from build123d import *

# Parameters (mm, degrees)
BOSS_EXTRUDE1_DEPTH = 97
FILLET1_R           = 3
SKETCH2_W           = 12.4
SKETCH2_H           = 5
CUT_EXTRUDE1_DEPTH  = 10


with BuildPart() as part:
    # Sketch1 → Boss-Extrude1 (new body)
    with BuildSketch(Plane(origin=(0, 0, 0), x_dir=(1, 0, 0), z_dir=(0, 1, 0))):
        with BuildLine():
            Line((-30, 11.1), (30, 11.1))
            ThreePointArc((30, 11.1), (37.071067812, 8.171067812), (40, 1.1))
            Line((40, 1.1), (40, -1.1))
            ThreePointArc((40, -1.1), (37.071067812, -8.171067812), (30, -11.1))
            Line((30, -11.1), (-30, -11.1))
            ThreePointArc((-30, -11.1), (-37.071067812, -8.171067812), (-40, -1.1))
            Line((-40, -1.1), (-40, 1.1))
            ThreePointArc((-40, 1.1), (-37.071067812, 8.171067812), (-30, 11.1))
        make_face()
    extrude(amount=BOSS_EXTRUDE1_DEPTH)

    # Fillet1
    fillet1_edges = [part.edges().sort_by_distance(p)[0] for p in [
        (37.071067812, 97, -8.171067812),
        (40, 0, 0),
        (37.071067812, 0, 8.171067812),
        (0, 97, -11.1),
        (-37.071067812, 97, -8.171067812),
        (-40, 97, 0),
        (-37.071067812, 97, 8.171067812),
        (0, 97, 11.1),
        (37.071067812, 97, 8.171067812),
        (40, 97, 0),
        (0, 0, 11.1),
        (-37.071067812, 0, 8.171067812),
        (-40, 0, 0),
        (-37.071067812, 0, -8.171067812),
        (0, 0, -11.1),
        (37.071067812, 0, -8.171067812),
    ]]
    fillet(fillet1_edges, radius=FILLET1_R)

    # Sketch2 → Cut-Extrude1 (cut)
    with BuildSketch(Plane(origin=(0, 97, 0), x_dir=(1, 0, 0), z_dir=(0, 1, 0))):
        with Locations((-24.3, 0)):
            Rectangle(SKETCH2_W, SKETCH2_H)
        with Locations((-4.2, 0)):
            Rectangle(SKETCH2_W, SKETCH2_H)
    extrude(amount=-CUT_EXTRUDE1_DEPTH, mode=Mode.SUBTRACT)


solid = part.part
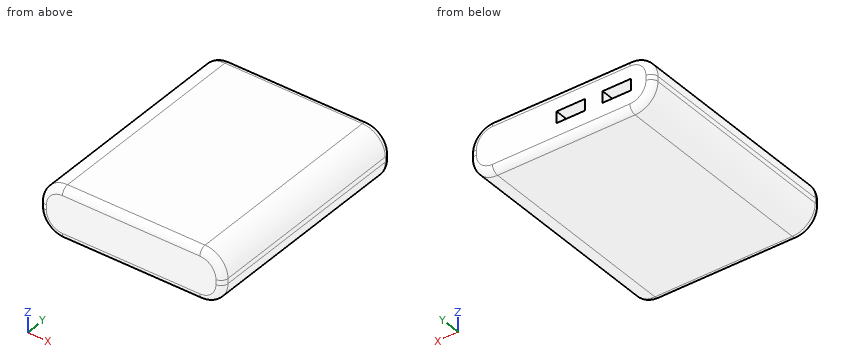
Build history of the part. All positions in model axes, mm. Coordinates: 2 decimals unless noted, no trailing zeros. Order: outer loops, then holes, each group sorted by start corner. A loop starts at its lowest first (then second) coordinate and runs counter-clockwise, first axis right, second up. Notation, with made-up numbers: (-37.5, 19) - (5.5, 19) arc R15 ccw to (5.5, 28) - close; hole circle Ø10 at (-31.75, -32). An arc over 180 degrees is marked (long way). Write each question's results on one line, items separated by ' | '. Start each with the question number.
Item 1: Band-saw the part on A-A on y = 88.5. Write the cut outline in (x, z), and give its area (3 significant figures).
Item 2: Band-saw the part on B-B on y = 40. Write the cut outline in (x, z), and give its area (3 significant figures).
Item 3: Flat gauge pins, fed straight in: pin 1 (12 mm diameter, centred on x = 22.5, z = -8.5, fed in from +Y); pin 2 (1.5 mm diameter, centred on x = -3.5, z = 0, fed in from +Y). Where does each tip first touch, or does it go through?
Item 4: Wall check: probe 1 along Y at (x, z) = (-9, 1); probe 2 along X at (y, z) = (15, -1.25); probe 3 along X at (y, z) = (72.5, 10.25). Give the ranges that are in metal, low to high. Write a range as [from, to].
Numbers:
1) outline: (-40, -1.1) arc R10 ccw to (-30, -11.1) - (30, -11.1) arc R10 ccw to (40, -1.1) - (40, 1.1) arc R10 ccw to (30, 11.1) - (-30, 11.1) arc R10 ccw to (-40, 1.1) - close; hole (-30.5, -2.5) - (-18.1, -2.5) - (-18.1, 2.5) - (-30.5, 2.5) - close; hole (-10.4, -2.5) - (2, -2.5) - (2, 2.5) - (-10.4, 2.5) - close | area: 1,570 mm^2
2) outline: (-40, -1.1) arc R10 ccw to (-30, -11.1) - (30, -11.1) arc R10 ccw to (40, -1.1) - (40, 1.1) arc R10 ccw to (30, 11.1) - (-30, 11.1) arc R10 ccw to (-40, 1.1) - close | area: 1,690 mm^2
3) pin 1: y = 97 | pin 2: y = 87
4) probe 1: [0, 87] | probe 2: [-40, 40] | probe 3: [-34.03, 34.03]
